The model under review builds one solid part; all positions refer to its coordinate system, in mm. A direction names the side the tool comes from. Coordinates: 2 decimals unless noted, no trailing zeros. Loops run counter-clockwise (first coordinate to the right, second up) from the corner with the lowest first, then second, coordinate; pieces in that order, holes last. Notation, with made-up numbers: M -38,-18.75 L -1,-18.75 A38 ccw -1,19.25 Z; hole C 12.5,-9.5 d1. An arc over 180 degrees is marked long. Return JSON: item names as keys, results as strings.
```python
from build123d import *

# Parameters (mm, degrees)
SKETCH1_R                 = 3.175
BOSS_EXTRUDE1_DEPTH       = 76.2
F_8_32_TAPPED_HOLE1_D     = 3.4544
F_8_32_TAPPED_HOLE1_DEPTH = 10
F_8_32_TAPPED_HOLE1_TIP   = 1.037806461
F_8_32_TAPPED_HOLE2_D     = 3.4544
F_8_32_TAPPED_HOLE2_DEPTH = 10
F_8_32_TAPPED_HOLE2_TIP   = 1.037806461


with BuildPart() as part:
    # Sketch1 → Boss-Extrude1 (new body)
    with BuildSketch(Plane(origin=(0, 0, 0), x_dir=(1, 0, 0), z_dir=(0, 1, 0))):
        with Locations(Location((0, 0, 0), (0, 0, 90))):
            Circle(SKETCH1_R)
    extrude(amount=BOSS_EXTRUDE1_DEPTH)

    # #8-32 Tapped Hole1
    with Locations(Plane(origin=(0, 76.2, 0), x_dir=(1, 0, 0), z_dir=(0, 1, 0))):
        with Locations((0, 0)):
            Hole(F_8_32_TAPPED_HOLE1_D / 2, depth=F_8_32_TAPPED_HOLE1_DEPTH)
            with Locations((0, 0, -(F_8_32_TAPPED_HOLE1_DEPTH + F_8_32_TAPPED_HOLE1_TIP / 2))):  # 118° drill point
                Cone(0, F_8_32_TAPPED_HOLE1_D / 2, F_8_32_TAPPED_HOLE1_TIP, mode=Mode.SUBTRACT)

    # #8-32 Tapped Hole2
    with Locations(Plane(origin=(0, 0, 0), x_dir=(-1, 0, 0), z_dir=(0, -1, 0))):
        with Locations((0, 0)):
            Hole(F_8_32_TAPPED_HOLE2_D / 2, depth=F_8_32_TAPPED_HOLE2_DEPTH)
            with Locations((0, 0, -(F_8_32_TAPPED_HOLE2_DEPTH + F_8_32_TAPPED_HOLE2_TIP / 2))):  # 118° drill point
                Cone(0, F_8_32_TAPPED_HOLE2_D / 2, F_8_32_TAPPED_HOLE2_TIP, mode=Mode.SUBTRACT)


solid = part.part
```
1. Add section A-A on y = 38. Give the boundary of the cut face in (x, z) (3 decimals), plus the area to 3 significant figures.
Check values:
{"outline": "C 0,0 d6.35", "area": "31.7 mm²"}
2. Insertion check: pin 1 Ø1.5 at (y, z) = (49.5, -2.5) entering from -X; pin 2 Ø3 at (x, z) = (0, 0) entering from -Y. Each pin has a flat end and moves straight along its axis. Give the tip position at first contact, or say it passes through.
Check values:
{"pin 1": "x = -2.65", "pin 2": "y = 10.14"}
3. The part is to be moulded in two halves that separate along X. For faces 3 (the face through (0.225, 71.13, -1.713)), 4 (the face through (1.93, 37.57, 2.52)), 5 (the face through (1.4, 76.2, -1.4)), say which applies: released by +X, released by -X, zero draft, split by the parting line, or undercut.
Check values:
{"face 3": "undercut", "face 4": "split by the parting line", "face 5": "zero draft"}
4. Machinability: for faces 1 (the face through (-0.225, 5.07, -1.713)), 2 (the face through (1.4, 0, -1.4)), which of the approach directions +Z, -Z, +X, -X, +Y, -Y give a long, thin tool a straight path to every point of the face, cutting with its end or side? Answer none if there is none.
Check values:
{"face 1": "-Y", "face 2": "+Z, -Z, +X, -X, -Y"}
5. Add section B-B on z = -2.5. Give the boundary of the cut face in (x, y).
Check values:
{"outline": "M -1.96,0 L 1.96,0 L 1.96,76.2 L -1.96,76.2 Z"}
6. To check wall thickness, follow line 1 (Z direction, x = 0.25, y = 45); line 2 (X direction, y = 67.5, z = 0.25). State the ranges of each line that lie inside material, in increasing order.
Check values:
{"line 1": "-3.17 to 3.17", "line 2": "-3.17 to -1.71, 1.71 to 3.17"}
7. Add section C-C on x = -2.5. Give the boundary of the cut face in (y, z), plus the area to 3 significant figures.
Check values:
{"outline": "M 0,-1.96 L 76.2,-1.96 L 76.2,1.96 L 0,1.96 Z", "area": "298 mm²"}
